Autodesk Inventor part; units mm, degrees
ref_plane "Work Plane1" through (6.5955, 0, -23.75) normal (-1, 0, 0) x (0, 1, 0)
ref_plane "YZ Plane" through (0, 0, 0) normal (1, 0, 0) x (0, 1, 0)
ref_plane "XZ Plane" through (0, 0, 0) normal (0, 1, 0) x (-1, 0, 0)
sketch "Sketch1" plane through (0, 0, 0) normal (0, 1, 0) x (-1, 0, 0)
  line L0 (-20, -20) -> (20, -20)
  line L1 (20, -20) -> (20, 20)
  line L2 (20, 20) -> (-20, 20)
  line L3 (-20, 20) -> (-20, -20)
  line L4 (-20, -20) -> (20, 20) construction
  line L5 (20, -20) -> (-20, 20) construction
  line L6 (20, 0) -> (25, 0)
  line L7 (25, 0) -> (25, 7.5)
  line L8 (20, 0) -> (20, 5)
  line L9 (20, 5) -> (25, 7.5)
  line L10 (25, 0) -> (25, -7.5)
  line L11 (20, 0) -> (20, -5)
  line L12 (20, -5) -> (25, -7.5)
  line L13 (0, -20) -> (5, -20)
  line L14 (0, -20) -> (-5, -20)
  line L15 (0, -20) -> (0, -25)
  line L16 (0, -25) -> (7.5, -25)
  line L17 (7.5, -25) -> (5, -20)
  line L18 (0, -25) -> (-7.5, -25)
  line L19 (-7.5, -25) -> (-5, -20)
  line L20 (-15, 0) -> (-15, -7.5)
  line L21 (-20, -5) -> (-15, -7.5)
  line L22 (-20, 0) -> (-15, 0)
  line L23 (-15, 0) -> (-15, 7.5)
  line L24 (-20, 5) -> (-15, 7.5)
  line L25 (-7.5, 15) -> (-5, 20)
  line L26 (0, 15) -> (-7.5, 15)
  line L27 (0, 20) -> (0, 15)
  line L28 (7.5, 15) -> (5, 20)
  line L29 (0, 15) -> (7.5, 15)
  line L30 (0, -24.75) -> (7.0955, -24.75)
  line L31 (7.0955, -24.75) -> (4.8455, -20.25)
  line L32 (4.8455, -20.25) -> (0, -20.25)
  line L33 (0, -24.75) -> (-7.0955, -24.75)
  line L34 (-7.0955, -24.75) -> (-4.8455, -20.25)
  line L35 (-4.8455, -20.25) -> (0, -20.25)
  line L36 (7.0955, -24.75) -> (4.7205, -20)
  line L37 (-7.0955, -24.75) -> (-4.7205, -20)
  line L38 (24.75, 0) -> (24.75, -7.0955)
  line L39 (24.75, -7.0955) -> (20.25, -4.8455)
  line L40 (20.25, -4.8455) -> (20.25, 0)
  line L41 (24.75, 0) -> (24.75, 7.0955)
  line L42 (24.75, 7.0955) -> (20.25, 4.8455)
  line L43 (20.25, 4.8455) -> (20.25, 0)
  line L44 (24.75, -7.0955) -> (20, -4.7205)
  line L45 (24.75, 7.0955) -> (20, 4.7205)
  line L46 (25, 0) -> (23.75, 0)
  line L47 (23.75, 0) -> (23.75, -6.875)
  line L48 (23.75, 0) -> (23.75, 6.875)
  line L49 (0, -25) -> (0, -23.75)
  line L50 (0, -23.75) -> (-6.875, -23.75)
  line L51 (0, -23.75) -> (6.875, -23.75)
  point P0 (0, 0)
  point P1 (-4.7205, -20)
  point P2 (4.7205, -20)
  point P3 (20, -4.7205)
  point P4 (20, 4.7205)
  point P5 (23.75, -6.5955)
  point P6 (23.75, 6.5955)
  point P7 (-6.5955, -23.75)
  point P8 (6.5955, -23.75)
  dimension "d0" = 40
  dimension "d1" = 40
  dimension "d2" = 5
  dimension "d3" = 7.5
  dimension "d4" = 5
  dimension "d5" = 7.5
  dimension "d6" = 5
  dimension "d7" = 5
  dimension "d8" = 5
  dimension "d9" = 5
  dimension "d10" = 7.5
  dimension "d11" = 7.5
  dimension "d14" = 40
  dimension "d21" = 40
  dimension "d43" = 0.25
  dimension "d44" = 0.25
  dimension "d45" = 0.25
  dimension "d46" = 0.25
  dimension "d56" = 1.25
  dimension "d57" = 1.25
extrude "Extrusion1" add sketch "Sketch1" along normal blind 30 contours L3 L21 L20 L23 L24 L2 L25 L26 L29 L28 L1 L0 | L0 L15 L35 L37 | L0 L36 L32 L15 | L35 L15 L50 L34 | L32 L31 L51 L15 | L1 L6 L40 L44 | L1 L45 L43 L6 | L40 L6 L47 L39 | L43 L42 L48 L6
sketch "Sketch2" plane through (0, 30, 0) normal (0, 1, 0) x (1, 0, 0)
  line L0 (-4.7205, 20) -> (-20, 20)
  line L1 (-20, 20) -> (0, 20)
  line L2 (0, 20) -> (0, 0)
  circle A0 centre (-10, 10) radius 5.5
  circle A1 centre (7.5, 10) radius 5.5
  circle A2 centre (-10, -7.5) radius 5.5
  circle A3 centre (7.5, -7.5) radius 5.5
  point P0 (-5, 20)
  dimension "d30" = 11
  dimension "d33" = 17.5
  dimension "d36" = 17.5
extrude "Extrusion2" cut sketch "Sketch2" against normal blind 25
fillet "Fillet1" radius 1 4 edges at (20, 15, -5) (20, 15, 5) (5, 15, 20) (-5, 15, 20)
fillet "Fillet2" radius 5 4 edges at (20, 15, -20) (20, 15, 20) (-20, 15, 20) (-20, 15, -20)
ref_plane "Work Plane1" through (6.5955, 0, -23.75) normal (-1, 0, 0) x (0, 1, 0)
sketch "Sketch3" plane through (6.5955, 0, -23.75) normal (-1, 0, 0) x (0, 1, 0)
  line L0 (0, -3.75) -> (30, -3.75)
  line L1 (15, -3.75) -> (15, 2)
  line L2 (0, 0) -> (5, 0)
  line L3 (15, 2) -> (15, -0.25)
  line L4 (15, 2) -> (15, 0.875)
  line L5 (30, -3.75) -> (30, 0)
  line L6 (25, 0) -> (30, 0)
  line L7 (0, 0) -> (30, 0)
  arc A0 (30, 0) -> (0, 0) centre (15, -55.25) ccw
  line L8 (15, 2) -> (15, 1)
  arc A1 (25, 0) -> (5, 0) centre (15, -49.5) ccw
  point P0 (0, -23.75)
  dimension "d48" = 5.75
  dimension "d55" = 5
  dimension "d60" = 1
  dimension "d61" = 5
extrude "Extrusion3" add sketch "Sketch3" along normal blind 13.191 contours L6 A1 L1 A0 | L1 A1 L2 A0
pattern_circular "Circular Pattern1" count 2 over 90 about axis through (0, 30, 0) along (0, 1, 0) of "Extrusion3"
fillet "Fillet3" radius 2 4 edges at (0, 30, -23.75) (0, 0, -23.75) (-23.75, 30, 0) (-23.75, 0, 0)
sketch "Sketch5" plane through (-6.5955, 0, -23.75) normal (-1, 0, 0) x (0, 0, 1)
  point P0 (23.75, 0)
properties part number "4x11mm_3DPrint"
Verification items for the finished model (mm, model axes). A direction names the side the tool comes from. Round coordinates to 2 decimals unless told otherwise and drop trailing zeros. Order: outer loops, then holes, each group sorted by start corner. A loop starts at its lowest first (then second) coordinate and runs counter-clockwise, first axis right, second up. Notation, with made-up numbers: (-33.75, 54) - (-16.75, 54) arc R12 ccw to (-16.75, 58) - close; hole circle Ø4 at (26.5, 40). An arc over 180 degrees is marked (long way). Use CSV: the item, a comma, the result in double quotes. Start each with the question number.
1) Section check D-D, the plane y = 20.5. State how many separate pieces and enclosed holes the cut face has, plus the area to 3 significant figures.
2) Thickness scan on L1, parallel to X at y = 24.75, z = -10; L2, parallel to Z at x = 8, y = 25.75; L3, parallel to Z at x = -6, y = 23.25. Record the ranges inside material, lowest first.
3) Mould release check, pull along X, two halves, no side actions. Record for faces 1 (the flat face through (-10, 5, 7)), 2 (the cylindrical face through (0.09, 14.81, -25.75)), 3 (the cylindrical face through (18, 15, 19)), 4 (the cylindrical face through (-18, 15, -19)): +X half, -X half, draft (parallel to the pull), parting line (faces both ways), or undercut.
4) Go/stop test with flat-tipped pins: P1, Ø3, axis at y = 12, z = 15, coming from the -X side; P2, Ø3.5, axis at x = -12, z = 5.5, coming from the +Y side; P3, Ø4, axis at y = 24, z = 6.5, coming from the -X side. Record where each tip stops, or that it passes through.
5) Section check A-A, the plane x = -2. Record the cut outline in (y, z), plus the area to 3 significant figures.
6) Access from +Z, -Z, +X, -X, +Y, -Y to the whole of each face (thin tool, end or side, straight path). Record for faces 5 (the flat face through (-25, 15, 6.596)), 6 (the flat face through (7, 5, 7)), 7 (the cylindrical face through (19.538, 15.21, 5.775)).
7) Section check B-B, the plane z = 0. Record the cut outline in (x, y), plus the area to 3 significant figures.
8) Section check C-C, the plane x = 17. Record the cut outline in (y, z), plus the area to 3 significant figures.
Answers:
1,separate pieces,"3"
1,enclosed holes,"4"
1,area,"1,180 mm²"
2,L1,"x = -20 to -15.5, -4.5 to 2, 13 to 20"
2,L2,"z = -20 to -15.48, -4.52 to 2.02, 12.98 to 20"
2,L3,"z = -25.15 to -24.07, -23.75 to -22.56, -20 to -13.77, -6.23 to 3.73, 11.27 to 15, 18 to 19.79"
3,face 1,"undercut"
3,face 2,"draft"
3,face 3,"+X half"
3,face 4,"-X half"
4,P1,"stops at x = -20"
4,P2,"stops at y = 5"
4,P3,"stops at x = -25.32"
5,outline,"(0, -22.2) arc R2 ccw to (1.53, -24.14) arc R57.25 ccw to (28.47, -24.14) arc R2 ccw to (30, -22.2) - (30, 15) - (0, 15) - close; hole (5, -23.75) arc R50.5 ccw to (25, -23.75) - close"
5,area,"1,190 mm²"
6,face 5,"+Z, -X, +Y, -Y"
6,face 6,"+Y"
6,face 7,"+Y, -Y"
7,outline,"(-24.14, 1.53) arc R2 ccw to (-22.2, 0) - (15, 0) - (15, 30) - (-22.2, 30) arc R2 ccw to (-24.14, 28.47) arc R57.25 ccw to start; hole (-23.75, 5) - (-23.75, 25) arc R50.5 ccw to start"
7,area,"1,190 mm²"
8,outline,"(0, -19.58) - (30, -19.58) - (30, -6.5) - (0, -6.5) - close; (0, 6.5) - (30, 6.5) - (30, 19.58) - (0, 19.58) - close"
8,area,"785 mm²"
